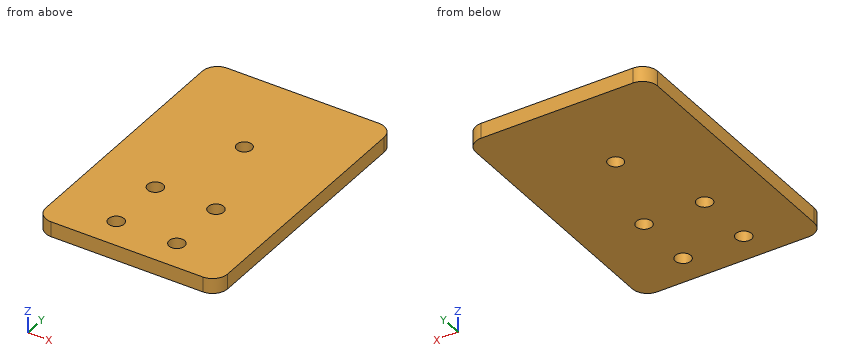
from build123d import *

# Parameters (mm, degrees)
SKETCH1_W      = 76.2
SKETCH1_H      = 114.3
SKETCH1_R      = 3.2639
SKETCH1_R_2    = 3.175
EXTRUDE1_DEPTH = 6.35
FILLET1_R      = 6.35


with BuildPart() as part:
    # Sketch1 → Extrude1 (new body)
    with BuildSketch(Plane.XY):
        with Locations((38.1, 57.15)):
            Rectangle(SKETCH1_W, SKETCH1_H)
        with Locations((25.4, 12.7)):
            Circle(SKETCH1_R, mode=Mode.SUBTRACT)
        with Locations((50.8, 12.7)):
            Circle(SKETCH1_R, mode=Mode.SUBTRACT)
        with Locations((25.4, 38.1)):
            Circle(SKETCH1_R, mode=Mode.SUBTRACT)
        with Locations((50.8, 38.1)):
            Circle(SKETCH1_R, mode=Mode.SUBTRACT)
        with Locations((38.1, 76.2)):
            Circle(SKETCH1_R_2, mode=Mode.SUBTRACT)
    extrude(amount=EXTRUDE1_DEPTH)

    # Fillet1
    fillet1_edges = [part.edges().sort_by_distance(p)[0] for p in [
        (0, 114.3, 3.175),
        (76.2, 114.3, 3.175),
        (76.2, 0, 3.175),
        (0, 0, 3.175),
    ]]
    fillet(fillet1_edges, radius=FILLET1_R)


solid = part.part
The model under review builds one solid part; all positions refer to its coordinate system, in mm. Round coordinates to 2 decimals unless told otherwise and drop trailing zeros. Loops run counter-clockwise (first coordinate to the right, second up) from the corner with the lowest first, then second, coordinate; pieces in that order, holes last. Notation, with made-up numbers: (17, -39) -> (25, -39) arc R17 cw to (25, -14) -> close; hole circle Ø8 at (35.5, 86.25). An arc over 180 degrees is marked (long way). One line per question, with ' | ' between items. Start each with the question number.
Item 1: Add section D-D, the plane x = 50.8. Write out the cut boundary in (y, z).
Item 2: Add section B-B, the plane y = 38.1. Write out the cut boundary in (x, z).
Item 3: Add section C-C, the plane z = 3.75. Write out the cut boundary in (x, y) (3 decimals).
Item 4: Wall thickness on line 1 along Y through (x, z) = (25.4, 4.25); line 2 along Y through (x, z) = (38.1, 2.25) (3 decimals); line 3 along X through (y, z) = (6, 3): over which ranges is each line inside the solid? List them lowest first. Write a range as [from, to].
Item 5: Add section A-A, the plane x = 38.1. Write out the cut boundary in (y, z) (3 decimals).
Return value:
1) outline: (0, 0) -> (9.44, 0) -> (9.44, 6.35) -> (0, 6.35) -> close; (15.96, 0) -> (34.84, 0) -> (34.84, 6.35) -> (15.96, 6.35) -> close; (41.36, 0) -> (114.3, 0) -> (114.3, 6.35) -> (41.36, 6.35) -> close
2) outline: (0, 0) -> (22.14, 0) -> (22.14, 6.35) -> (0, 6.35) -> close; (28.66, 0) -> (47.54, 0) -> (47.54, 6.35) -> (28.66, 6.35) -> close; (54.06, 0) -> (76.2, 0) -> (76.2, 6.35) -> (54.06, 6.35) -> close
3) outline: (0, 6.35) arc R6.35 ccw to (6.35, 0) -> (69.85, 0) arc R6.35 ccw to (76.2, 6.35) -> (76.2, 107.95) arc R6.35 ccw to (69.85, 114.3) -> (6.35, 114.3) arc R6.35 ccw to (0, 107.95) -> close; hole circle Ø6.528 at (25.4, 12.7); hole circle Ø6.528 at (25.4, 38.1); hole circle Ø6.35 at (38.1, 76.2); hole circle Ø6.528 at (50.8, 12.7); hole circle Ø6.528 at (50.8, 38.1)
4) line 1: y = [0, 9.44], [15.96, 34.84], [41.36, 114.3] | line 2: y = [0, 73.025], [79.375, 114.3] | line 3: x = [0.01, 76.19]
5) outline: (0, 0) -> (73.025, 0) -> (73.025, 6.35) -> (0, 6.35) -> close; (79.375, 0) -> (114.3, 0) -> (114.3, 6.35) -> (79.375, 6.35) -> close
